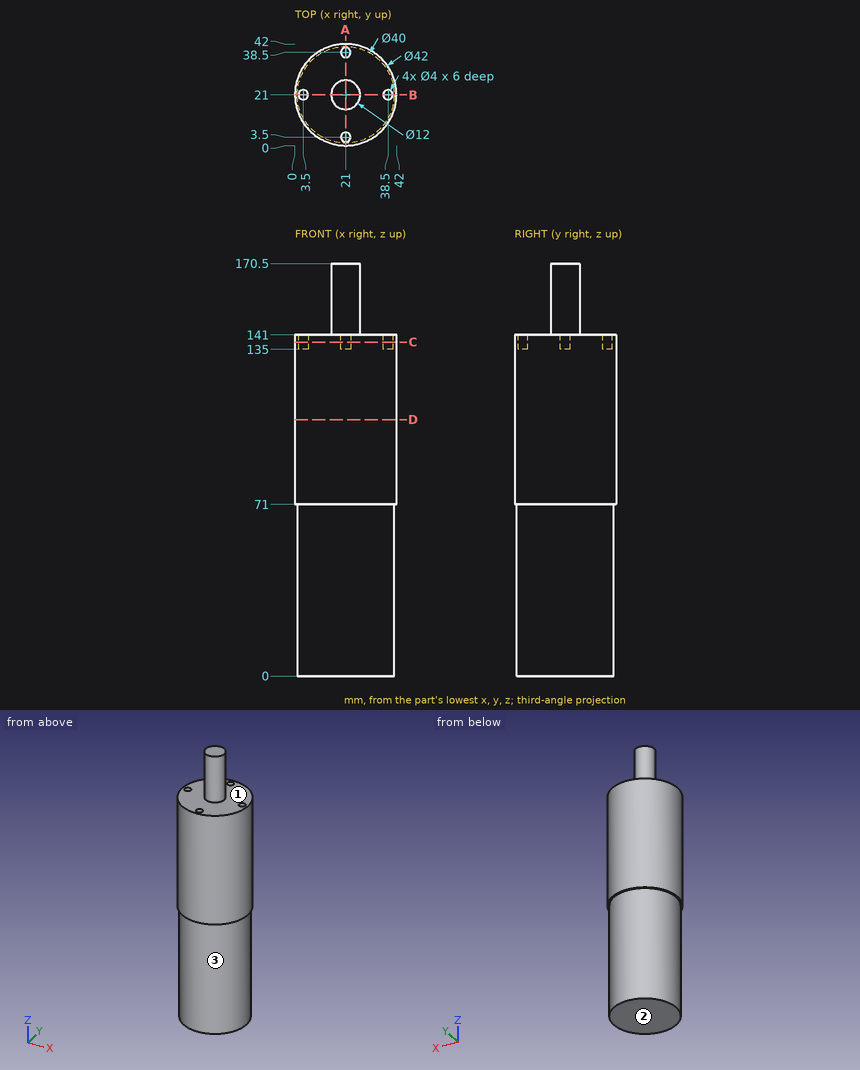
Part print with two shaded views. Sizes in mm from the minimum x, y, z corner. A direction names the side the tool comes from. Coordinates: 2 decimals unless noted, no trailing zeros. Order: outer loops, then holes, each group sorted by start corner. A loop starts at its lowest first (then second) coordinate and runs counter-clockwise, first axis right, second up. Notation, with made-up numbers: M -7,38 L 17,38 A20 ccw 17,68 Z; hole C 32,82 d10. An arc over 180 degrees is marked long. Use a Markdown table: item, result.
(1) Cut at A-A on x = 21. Write the cut outline in (y, z), then the cut area to 3 significant figures.
A:
| item | result |
|---|---|
| outline | M 0,71 L 1,71 L 1,0 L 41,0 L 41,71 L 42,71 L 42,141 L 40.5,141 L 40.5,135 L 36.5,135 L 36.5,141 L 27,141 L 27,170.5 L 15,170.5 L 15,141 L 5.5,141 L 5.5,135 L 1.5,135 L 1.5,141 L 0,141 Z |
| area | 6,090 mm^2 |
(2) Flat gauge pins, fed straight in: pin 1 (6 mm diameter, centred on y = 8.5, z = 102.5, fed in from +X); pin 2 (3 mm diameter, centred on y = 5, z = 102, fed in from +X); pin 3 (5 mm diameter, centred on x = 21, y = 3.5, fed in from +Z). Where does each tip first touch, or does it go through?
A:
| item | result |
|---|---|
| pin 1 | stops at x = 39.73 |
| pin 2 | stops at x = 36.19 |
| pin 3 | stops at z = 141 |
(3) Cut at D-D on z = 106. Write the cut outline in (x, y).
A:
| item | result |
|---|---|
| outline | C 21,21 d42 |
(4) Cut at C-C on z = 138. Write the cut outline in (x, y), then the cut area to 3 significant figures.
A:
| item | result |
|---|---|
| outline | C 21,21 d42; hole C 3.5,21 d4; hole C 21,3.5 d4; hole C 21,38.5 d4; hole C 38.5,21 d4 |
| area | 1,340 mm^2 |
(5) Probe L1, parallel to Y at x = 21, z = 139.3; L2, parallel to Z at x = 26.5, y = 5; L3, parallel to X at y = 21.5, z = 86. List the from-to ranges inside material, lowest first.
A:
| item | result |
|---|---|
| L1 | y = 0 to 1.5, 5.5 to 36.5, 40.5 to 42 |
| L2 | z = 0 to 141 |
| L3 | x = 0.01 to 41.99 |
(6) Tool access for the marked faces 1, 2 and 3: list every direction of +Z, -Z, +X, -X, +Y, -Y with a clear straight run to the whole face (end or side of a thin tool).
A:
| item | result |
|---|---|
| face 1 | +Z |
| face 2 | -Z, +X, -X, +Y, -Y |
| face 3 | -Z |
